```python
from build123d import *

# Parameters (mm, degrees)
FILLET1_R = 3
FILLET2_R = 7


with BuildPart() as part:
    # Sketch1 → Revolve1 (revolve)
    with BuildSketch(Plane.XY):
        Polygon((0, 0), (0, 21), (37, 21), (37, 8), (97, 8), (97, 0), align=None)
    revolve(axis=Axis((97, 0, 0), (-1, 0, 0)))

    # Fillet1
    fillet1_edges = [part.edges().sort_by_distance(p)[0] for p in [
        (37, -21, 0),
    ]]
    fillet(fillet1_edges, radius=FILLET1_R)

    # Fillet2
    fillet2_edges = [part.edges().sort_by_distance(p)[0] for p in [
        (37, -8, 0),
    ]]
    fillet(fillet2_edges, radius=FILLET2_R)


solid = part.part
```
Source: CAD feature listing. Evaluate the final solid. Frame: model axes, mm. A direction names the side the tool comes from. Give positions to 0.01 mm unless a question says otherwise; leave off trailing zeros. Loops run counter-clockwise (first coordinate to the right, second up) from the corner with the lowest first, then second, coordinate; pieces in that order, holes last. Notation, with made-up numbers: (-0.75, 5) - (7.25, 5) arc R19 ccw to (7.25, 11) - close; hole circle Ø10 at (80, -21). An arc over 180 degrees is marked (long way). Use CSV: the item, a comma, the result in double quotes.
1) Cut plane A-A (z = 0). Output: boundary loops of the cut face in (x, y), and give its area (3 significant figures).
Worked out:
outline,"(0, -21) - (34, -21) arc R3 ccw to (37, -18) - (37, -15) arc R7 cw to (44, -8) - (97, -8) - (97, 8) - (44, 8) arc R7 cw to (37, 15) - (37, 18) arc R3 ccw to (34, 21) - (0, 21) - close"
area,"2,530 mm^2"
2) Cut plane C-C (x = 45). Output: boundary loops of the cut face in (y, z), and give its area (3 significant figures).
Worked out:
outline,"circle Ø16 at (0, 0)"
area,"201 mm^2"
3) Set-up query: faces 1 (the cylindrical face through (70.87, -1.73, 7.81)), 2 (the cylindrical face through (17.24, 20.03, -6.31)). Return all of +Z, -Z, +X, -X, +Y, -Y with unobstructed straight access to the full face (end or side cutting, diameter ignored); none if empty.
Worked out:
face 1,"+X"
face 2,"+X, -X"
4) Pin query (flat end, axial travel): P1, Ø1, axis at y = -10, z = -6.5, coming from the +X side; P2, Ø3, axis at x = 34.5, y = -10.5, coming from the -Z side; P3, Ø1, axis at x = 49.5, y = 0, coming from the +Z side; P4, Ø3, axis at y = 7, z = 8.5, coming from the -X side. Return the tip coordinate at first contact, or that it passes through.
Worked out:
P1,"stops at x = 37.98"
P2,"stops at z = -18.95"
P3,"stops at z = 8"
P4,"stops at x = 0"
5) Line query: line 1 (X direction, y = 10.5, z = 11); line 2 (Z direction, x = 18.5, y = 0.5); line 3 (Y direction, x = 10, z = 9). Output: solid intervals per line, ascending.
Worked out:
line 1,"x = 0 to 37"
line 2,"z = -20.99 to 20.99"
line 3,"y = -18.97 to 18.97"
